Autodesk Inventor part; units mm, degrees
ref_plane "Work Plane3" through (-4.3301, 20, -20) normal (0, 1, 0) x (1, 0, 0)
ref_plane "Work Plane2" through (0, 21.5, 0) normal (0, 1, 0) x (1, 0, 0)
ref_plane "YZ Plane" through (0, 0, 0) normal (1, 0, 0) x (0, 1, 0)
ref_plane "Work Plane3" through (-4.3301, 20, -20) normal (0, 1, 0) x (1, 0, 0)
sketch "Sketch4" plane through (-4.3301, 20, -20) normal (0, 1, 0) x (1, 0, 0)
  circle A0 centre (4.3301, -20) radius 50
  dimension "d16" = 100
extrude "Extrusion4" add sketch "Sketch4" along normal blind 1.5
sketch "Sketch9" plane through (0, 0, 0) normal (0, 0, 1) x (1, 0, 0)
  line L0 (50, 21.5) -> (-50, 21.5)
  line L1 (50, 21.5) -> (43, 21.5)
  line L2 (50, 21.5) -> (50, 26.5)
  line L3 (50, 26.5) -> (48, 26.5)
  line L4 (48, 26.5) -> (43, 21.5)
  line L5 (0, 21.5) -> (0, 37.2)
  point P0 (0, 0)
  dimension "d27" = 7
  dimension "d28" = 5
  dimension "d29" = 2
revolve "Revolution1" add sketch "Sketch9" angle 360 about axis through (0, 21.5, 0) along (0, 1, 0)
ref_plane "Work Plane2" through (0, 21.5, 0) normal (0, 1, 0) x (1, 0, 0)
sketch "Sketch12" plane through (0, 21.5, 0) normal (0, 1, 0) x (1, 0, 0)
  line L0 (0, 0) -> (20, 0)
  line L1 (20, 0) -> (20, -30)
  line L2 (20, -30) -> (-20, -30)
  line L3 (-20, -30) -> (-20, 30)
  line L4 (-20, 30) -> (20, 30)
  line L5 (20, 30) -> (20, -30)
  circle A0 centre (20, 30) radius 1.75
  circle A1 centre (-20, 30) radius 1.75
  circle A2 centre (-20, -30) radius 1.75
  circle A3 centre (20, -30) radius 1.75
  dimension "d47" = 20
  dimension "d48" = 30
  dimension "d49" = 40
  dimension "d50" = 60
  dimension "d51" = 3.5
  dimension "d52" = 3.5
  dimension "d53" = 3.5
  dimension "d54" = 3.5
extrude "Extrusion6" cut sketch "Sketch12" against normal blind 1.5 contours A3 L2 L1 | L1 L2 A3 | A0 L4 L5 | L5 L4 A0 | A2 L3 L2 | L2 L3 A2 | A1 L3 L4 | L4 L3 A1
sketch "Sketch13" plane through (0, 0, 0) normal (0, 0, 1) x (1, 0, 0)
  line L0 (0, 0) -> (25, 0) construction
  line L1 (-50, 20) -> (50, 20)
  line L2 (0, 7.5) -> (-21.6506, 20)
  line L3 (0, 7.5) -> (21.6506, 20)
  line L4 (0, 7.5) -> (25, 7.5) construction
  line L5 (21.6506, 20) -> (-21.6506, 20)
  line L6 (0, 7.5) -> (0, 12.5)
  line L7 (0, 20) -> (-5, 20)
  line L8 (-5, 20) -> (0, 12.5)
  line L9 (0, 20) -> (5, 20)
  line L10 (5, 20) -> (0, 12.5)
  dimension "d60" = 25
  dimension "d61" = 30
  dimension "d62" = 5
  dimension "d63" = 5
  dimension "d64" = 5
extrude "Extrusion7" add sketch "Sketch13" along normal mid plane 40 contours L1 L8 L6 L2 | L6 L10 L1 L3
sketch "Sketch16" plane through (0, 0, 20) normal (0, 0, 1) x (1, 0, 0)
  line L0 (-50, 20) -> (50, 20)
  line L1 (0, 20) -> (0, 5)
  line L2 (0, 5) -> (23.8952, 18.7959)
  line L3 (23.8952, 18.7959) -> (25.9808, 20)
  line L4 (25.9808, 20) -> (-25.9812, 20)
  line L5 (-25.9812, 20) -> (0, 5)
  point P0 (0, 0)
  dimension "d67" = 15
  dimension "d68" = 60
  dimension "d69" = 51.962
extrude "Extrusion8" add sketch "Sketch16" against normal blind 40
sketch "Sketch17" plane through (0, 0, 20) normal (0, 0, 1) x (1, 0, 0)
  line L0 (0, 5) -> (-25.9812, 20)
  line L1 (0, 5) -> (0, 10)
  line L2 (0, 10) -> (6.8298, 16.8298)
  line L3 (6.8298, 16.8298) -> (10, 20)
  line L4 (-50, 20) -> (50, 20)
  line L5 (10, 20) -> (-10, 20)
  line L6 (-10, 20) -> (0, 10)
  point P0 (0, 0)
  dimension "d72" = 5
  dimension "d73" = 135
  dimension "d74" = 20
extrude "Extrusion9" cut sketch "Sketch17" against normal blind 40 contours L6 L4 L3 L2
sketch "Sketch18" plane through (0, 20, 0) normal (0, -1, 0) x (1, 0, 0)
  line L0 (0, 0) -> (-35.3553, 35.3553)
  circle A0 centre (0, 0) radius 50
  line L1 (0, 0) -> (50, 0) construction
  line L2 (0, 0) -> (35.3553, 35.3553)
  line L3 (0, 0) -> (50, 0) construction
  line L4 (0, 0) -> (-35.3553, -35.3553)
  line L5 (0, 0) -> (50, 0) construction
  line L6 (0, 0) -> (35.3553, -35.3553)
  line L7 (0, 0) -> (50, 0) construction
  circle A1 centre (0, 0) radius 43
  line L8 (-30.4056, 30.4056) -> (-29.3449, 29.3449)
  line L9 (30.4056, 30.4056) -> (29.3449, 29.3449)
  line L10 (30.4056, -30.4056) -> (29.3449, -29.3449)
  line L11 (-30.4056, -30.4056) -> (-29.3449, -29.3449)
  circle A2 centre (-29.3449, -29.3449) radius 1.5
  circle A3 centre (29.3449, -29.3449) radius 1.5
  circle A4 centre (-29.3449, 29.3449) radius 1.5
  circle A5 centre (29.3449, 29.3449) radius 1.5
  dimension "d77" = 135
  dimension "d78" = 45
  dimension "d79" = 135
  dimension "d80" = 45
  dimension "d81" = 1.5
  dimension "d82" = 1.5
  dimension "d83" = 1.5
  dimension "d84" = 1.5
extrude "Extrusion10" cut sketch "Sketch18" against normal blind 40 contours A4 L0 | L0 A4 | A5 L2 | L2 A5 | A2 L4 | L4 A2 | A3 L6 | L6 A3
properties part number "Mirror Mount" material "Acetal Resin, Black"
Input: part model. Units: mm. Frame: model coordinates. A direction names the side the tool comes from. Give positions to 0.01 mm unless a question says otherwise; leave off trailing zeros. Write each loop counter-clockwise with the first axis right and the second up, starting at its lowest first coordinate (ties: lowest second). Pieces come first, ordered by that corner, then holes.
Q1. First-contact query: P1, Ø3, axis at x = 20, z = 30, coming from the -Y side; P2, Ø1.5, axis at x = -23.5, y = 20, coming from the +Z side; P3, Ø4, axis at y = 22.5, z = 12, coming from the -X side; P4, Ø2, axis at x = -12, y = 11, coming from the +Z side. Flat tips, straight axial feed; report the tip coordinate or a pass-through.
Q2. Set-up query: faces 5 (the face through (0, 9, -20)), 6 (the face through (0, 9, 20)), 7 (the face through (5, 15, 0)). Return all of +Z, -Z, +X, -X, +Y, -Y with unobstructed straight access to the full face (end or side cutting, diameter ignored); none if empty.
Q3. Section A-A, the plane z = 0. Output: boundary loops of the cut face in (x, y), plus the area to 3 significant figures.
Q4. Material intervals for probe 1 along X at (y, z) = (20.4, -30); probe 2 along Z at (x, y) = (20, 21.1); probe 3 along Y at (x, z) = (37.5, 8.5), sorted ascending.
Q5. Section C-C, the plane x = 20.5. State how many separate pieces and enclosed holes the cut face has, plus the area to 3 significant figures.
Q6. Pull-direction query (Y, two-part tool) for faces 1 (the face through (-5, 15, 0)), 2 (the face through (-21.39, 20.76, 31.06)), 3 (the face through (-1, 21.5, -1)), 4 (the face through (-13.172, 12.605, 0.28)); classes: pulls with the +Y half, pulls with the -Y half, needs draft (parallel to the pull), parting line crosses it, or undercut.
Q7. Section B-B, the plane y = 13.5. Output: boundary loops of the cut face in (x, z).
Filled in:
1. P1: passes through
1. P2: stops at z = 44.52
1. P3: stops at x = -48.99
1. P4: stops at z = 20
2. face 5: -Z, +X, -X, -Y
2. face 6: +Z, +X, -X, -Y
2. face 7: +Z, -Z
3. outline: (-50, 20) - (-25.98, 20) - (0, 5) - (23.9, 18.8) - (25.98, 20) - (50, 20) - (50, 26.5) - (48, 26.5) - (43, 21.5) - (-43, 21.5) - (-48, 26.5) - (-50, 26.5) - close; hole (-10, 20) - (0, 10) - (10, 20) - close
3. area: 485 mm2
4. probe 1: x = -40 to -30.69, -28 to -21.75, -18.25 to 18.25, 21.75 to 28, 30.69 to 40
4. probe 2: z = -45.83 to -31.75, -28.25 to 28.25, 31.75 to 45.83
4. probe 3: y = 20 to 21.5
5. separate pieces: 3
5. enclosed holes: 0
5. area: 303 mm2
6. face 1: undercut
6. face 2: needs draft
6. face 3: pulls with the +Y half
6. face 4: pulls with the -Y half
7. outline: (-14.72, -20) - (-3.5, -20) - (-3.5, 20) - (-14.72, 20) - close; (3.5, -20) - (14.72, -20) - (14.72, 20) - (3.5, 20) - close
